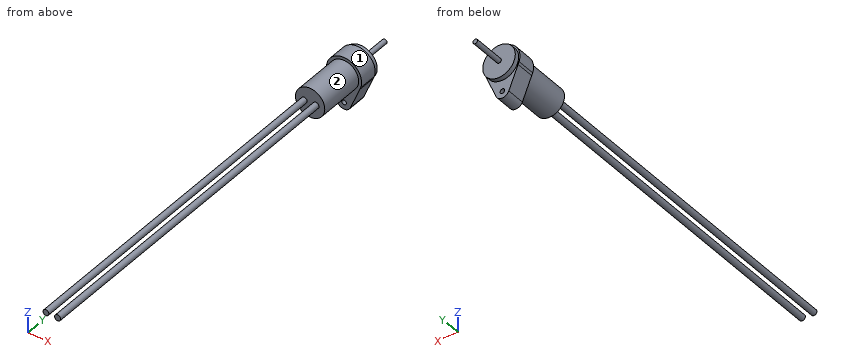
```python
from build123d import *

# Parameters (mm, degrees)
F0_R     = 3.175
F1_DEPTH = 15
F2_R     = 0.5
F3_DEPTH = 7
F4_R     = 0.5
F4_R_2   = 3.175
F5_DEPTH = 5
F6_R     = 9.3189524644
F6_R_2   = 3.5292713956
F7_DEPTH = 1
F8_R     = 0.635
F8_R_2   = 0.6612583991
F9_DEPTH = 76.2


with BuildPart() as f1:
    # F0 (on Front) → F1 (new body)
    with BuildSketch(Plane.XZ):
        Circle(F0_R)
    extrude(amount=F1_DEPTH)

    # F2 (on face) → F3 (join)
    with BuildSketch(Plane(origin=(0, 0, 0), x_dir=(-1, 0, 0), z_dir=(0, 1, 0))):
        Circle(F2_R)
    extrude(amount=F3_DEPTH)

    # F4 (on face) → F5 (join)
    with BuildSketch(Plane(origin=(0, 0, 0), x_dir=(-1, 0, 0), z_dir=(0, 1, 0))):
        with BuildLine():
            Line((1.3866466063, -6.6022387167), (3.4052943148, -1.7088214153))
            Line((3.4052943148, -1.7088214153), (3.6196746552, -1.1891406101))
            ThreePointArc((3.6196746552, -1.1891406101), (0, 3.81), (-3.6196746552, -1.1891406101))
            Line((-3.6196746552, -1.1891406101), (-3.4052943148, -1.7088214153))
            Line((-3.4052943148, -1.7088214153), (-1.3866466063, -6.6022387167))
            ThreePointArc((-1.3866466063, -6.6022387167), (0, -7.5302149504), (1.3866466063, -6.6022387167))
        make_face()
        with Locations((0, -6.0302149504)):
            Circle(F4_R, mode=Mode.SUBTRACT)
        Circle(F4_R_2, mode=Mode.SUBTRACT)
        Circle(F4_R_2)
        Circle(F4_R, mode=Mode.SUBTRACT)
    extrude(amount=-F5_DEPTH)

    # F6 (on face) → F7 (cut)
    with BuildSketch(Plane(origin=(0, 0, 0), x_dir=(-1, 0, 0), z_dir=(0, 1, 0))):
        Circle(F6_R)
        with Locations((0, -0.1206563757)):
            Circle(F6_R_2, mode=Mode.SUBTRACT)
    extrude(amount=-F7_DEPTH, mode=Mode.SUBTRACT)

    # F8 (on face) → F9 (join)
    with BuildSketch(Plane.XZ.offset(15)):
        with Locations((-1.27, 0)):
            Circle(F8_R)
        with Locations((1.27, 0)):
            Circle(F8_R_2)
    extrude(amount=F9_DEPTH)


solid = f1.part
```
Work out the finished part from the listing and answer in its coordinate system (mm). Face numbers are marked on the shaded views. A direction names the side the tool comes from. Coordinates: 2 decimals unless noted, no trailing zeros. Write each loop counter-clockwise with the first axis right and the second up, starting at its lowest first coordinate (ties: lowest second). Pieces come first, ordered by that corner, then holes.
Q1. Find the intervals of material crossed by line 1 (Y direction, x = -2.5, z = -1.5); line 2 (Y direction, x = 3, z = -1.75); line 3 (X direction, y = -3.5, z = -5), in increasing order.
Q2. Which of the six approach directions +Z, -Z, +X, -X, +Y, -Y give full straight-line access (tool end or side, diameter ignored) to the marked faces 1 and 2?
Q3. Each of these flat-tipped pins is pushed along its axis until it touches: pin 1 Ø3 at (y, z) = (-56.5, 2) entering from +X; pin 2 Ø2.5 at (x, z) = (0.5, -2.5) entering from +Y; pin 3 Ø1.5 at (x, y) = (-2, -12.5) entering from +Z. Where does it stop, or does it pass through?
Q4. A cutting plane is placed at B-B, the plane y = -7. Give the vertices of the cut face in (x, z) (3 decimals).
Q5. A cutting plane is placed at A-A, the plane y = -61. Give the vertices of the cut face in (x, z) (3 decimals).
Findings below:
1. line 1: y = -15 to 0
1. line 2: y = -5 to 0
1. line 3: x = -2.05 to 2.05
2. face 1: +Y, -Y
2. face 2: -Y
3. pin 1: stops at x = 1.7
3. pin 2: stops at y = 0
3. pin 3: stops at z = 2.92
4. outline: circle Ø6.35 at (0, 0)
5. outline: circle Ø1.27 at (-1.27, 0); circle Ø1.323 at (1.27, 0)
